from build123d import *

# Parameters (mm, degrees)
SKETCH1_R           = 1.513948887
SKETCH1_R_2         = 2.25
BOSS_EXTRUDE1_DEPTH = 2
SCALE1_SCALE        = 2.8


with BuildPart() as part:
    # Sketch1 → Boss-Extrude1 (new body)
    with BuildSketch(Plane.XY):
        with BuildLine():
            Line((-137.330840139, 84.740646997), (-129.065622639, 84.500215059))
            Line((-129.065622639, 84.500215059), (-129.094489584, 83.519353553))
            add(Edge.make_bspline(
                [(-129.094489584, 83.519353553), (-129.101127466, 83.291204798), (-129.199889222, 82.884598348), (-129.259340655, 82.689308143)],
                knots=[0.212765957, 0.212765957, 0.212765957, 0.212765957, 0.234042553, 0.234042553, 0.234042553, 0.234042553], degree=3))
            add(Edge.make_bspline(
                [(-129.259340655, 82.689308143), (-130.523557303, 78.537033893), (-136.295329969, 80.981325314), (-144.988370325, 77.341015795)],
                knots=[0.234042553, 0.234042553, 0.234042553, 0.234042553, 0.255319149, 0.255319149, 0.255319149, 0.255319149], degree=3))
            add(Edge.make_bspline(
                [(-144.988370325, 77.341015795), (-145.098029788, 77.295108948), (-145.047490899, 77.331606959), (-145.163209238, 77.309852904)],
                knots=[0.255319149, 0.255319149, 0.255319149, 0.255319149, 0.276595745, 0.276595745, 0.276595745, 0.276595745], degree=3))
            add(Edge.make_bspline(
                [(-145.163209238, 77.309852904), (-145.220654832, 77.299037913), (-145.285896319, 77.302718732), (-145.330562439, 77.26739941)],
                knots=[0.276595745, 0.276595745, 0.276595745, 0.276595745, 0.29787234, 0.29787234, 0.29787234, 0.29787234], degree=3))
            add(Edge.make_bspline(
                [(-145.330562439, 77.26739941), (-145.851667181, 76.854361866), (-147.089249586, 75.848112745), (-149.250531504, 76.047683454)],
                knots=[0.29787234, 0.29787234, 0.29787234, 0.29787234, 0.319148936, 0.319148936, 0.319148936, 0.319148936], degree=3))
            add(Edge.make_bspline(
                [(-149.250531504, 76.047683454), (-149.579241067, 76.078019194), (-149.46315051, 76.145142448), (-149.823167715, 76.007773448)],
                knots=[0.319148936, 0.319148936, 0.319148936, 0.319148936, 0.340425532, 0.340425532, 0.340425532, 0.340425532], degree=3))
            add(Edge.make_bspline(
                [(-149.823167715, 76.007773448), (-150.230952854, 75.852269176), (-150.642170668, 75.684998689), (-151.060274508, 75.505196874)],
                knots=[0.340425532, 0.340425532, 0.340425532, 0.340425532, 0.361702128, 0.361702128, 0.361702128, 0.361702128], degree=3))
            add(Edge.make_bspline(
                [(-151.060274508, 75.505196874), (-151.574575938, 75.284016862), (-153.203689978, 76.198038715), (-153.745700946, 75.937300235)],
                knots=[0.361702128, 0.361702128, 0.361702128, 0.361702128, 0.382978723, 0.382978723, 0.382978723, 0.382978723], degree=3))
            add(Edge.make_bspline(
                [(-153.745700946, 75.937300235), (-155.594836987, 75.047762033), (-159.716630745, 73.288289093), (-162.232470675, 71.858787121)],
                knots=[0.382978723, 0.382978723, 0.382978723, 0.382978723, 0.404255319, 0.404255319, 0.404255319, 0.404255319], degree=3))
            add(Edge.make_bspline(
                [(-162.232470675, 71.858787121), (-162.860836143, 71.501768336), (-162.462583912, 70.287097997), (-163.071821528, 69.816015174)],
                knots=[0.404255319, 0.404255319, 0.404255319, 0.404255319, 0.425531915, 0.425531915, 0.425531915, 0.425531915], degree=3))
            add(Edge.make_bspline(
                [(-163.071821528, 69.816015174), (-163.094733593, 69.798293477), (-163.120271861, 69.783446128), (-163.145313839, 69.766923799)],
                knots=[0.425531915, 0.425531915, 0.425531915, 0.425531915, 0.446808511, 0.446808511, 0.446808511, 0.446808511], degree=3))
            Line((-163.145313839, 69.766923799), (-163.880340349, 69.282192995))
            add(Edge.make_bspline(
                [(-163.880340349, 69.282192995), (-164.468258164, 68.894466252), (-164.620846731, 69.006028161), (-165.195757605, 69.192653966)],
                knots=[0.468085106, 0.468085106, 0.468085106, 0.468085106, 0.489361702, 0.489361702, 0.489361702, 0.489361702], degree=3))
            add(Edge.make_bspline(
                [(-165.195757605, 69.192653966), (-165.880330422, 69.414858475), (-166.586588499, 69.876830428), (-166.216843664, 70.149863853)],
                knots=[0.489361702, 0.489361702, 0.489361702, 0.489361702, 0.509556789, 0.509556789, 0.509556789, 0.509556789], degree=3))
            ThreePointArc((-166.216843664, 70.149863853), (-169.932333673, 71.346005011), (-168.915752591, 75.114583334))
            Line((-168.915752591, 75.114583334), (-169.065622639, 75.20554687))
            Line((-169.065622639, 75.20554687), (-169.064671417, 75.244319545))
            Line((-169.064671417, 75.244319545), (-169.037168666, 76.350054178))
            add(Edge.make_bspline(
                [(-169.037168666, 76.350054178), (-169.033053593, 76.794047826), (-168.700084206, 77.078711631), (-168.409216773, 77.250221263)],
                knots=[0.957446809, 0.957446809, 0.957446809, 0.957446809, 1, 1, 1, 1], degree=3))
            add(Edge.make_bspline(
                [(-168.409216773, 77.250221263), (-167.016522993, 78.071374807), (-166.193859899, 78.40091152), (-164.934151222, 79.073281388)],
                knots=[0, 0, 0, 0, 0.021276596, 0.021276596, 0.021276596, 0.021276596], degree=3))
            add(Edge.make_bspline(
                [(-164.934151222, 79.073281388), (-164.508106737, 79.300665029), (-163.405349845, 79.062094179), (-162.816253342, 79.349694368)],
                knots=[0.021276596, 0.021276596, 0.021276596, 0.021276596, 0.042553191, 0.042553191, 0.042553191, 0.042553191], degree=3))
            add(Edge.make_bspline(
                [(-162.816253342, 79.349694368), (-160.762294186, 80.3524281), (-156.1821764, 82.606350861), (-154.813800841, 83.397685633)],
                knots=[0.042553191, 0.042553191, 0.042553191, 0.042553191, 0.063829787, 0.063829787, 0.063829787, 0.063829787], degree=3))
            add(Edge.make_bspline(
                [(-154.813800841, 83.397685633), (-154.362548949, 83.658651579), (-154.360419036, 84.858143709), (-153.955446208, 85.0823635)],
                knots=[0.063829787, 0.063829787, 0.063829787, 0.063829787, 0.085106383, 0.085106383, 0.085106383, 0.085106383], degree=3))
            add(Edge.make_bspline(
                [(-153.955446208, 85.0823635), (-151.58212429, 86.396519351), (-151.052789401, 86.655893033), (-149.40636724, 86.835736205)],
                knots=[0.085106383, 0.085106383, 0.085106383, 0.085106383, 0.106382979, 0.106382979, 0.106382979, 0.106382979], degree=3))
            add(Edge.make_bspline(
                [(-149.40636724, 86.835736205), (-148.241325924, 86.963034649), (-146.873012401, 86.919588575), (-145.02819822, 86.765759283)],
                knots=[0.106382979, 0.106382979, 0.106382979, 0.106382979, 0.127659574, 0.127659574, 0.127659574, 0.127659574], degree=3))
            add(Edge.make_bspline(
                [(-145.02819822, 86.765759283), (-143.567802181, 86.644002746), (-141.759858228, 86.186588584), (-139.486373361, 85.727582157)],
                knots=[0.127659574, 0.127659574, 0.127659574, 0.127659574, 0.14893617, 0.14893617, 0.14893617, 0.14893617], degree=3))
            add(Edge.make_bspline(
                [(-139.486373361, 85.727582157), (-138.947939819, 85.618873917), (-138.058442974, 84.761801368), (-137.330840139, 84.740646997)],
                knots=[0.14893617, 0.14893617, 0.14893617, 0.14893617, 0.170212766, 0.170212766, 0.170212766, 0.170212766], degree=3))
        make_face()
        with Locations((-148.728458674, 81.356006962)):
            Circle(SKETCH1_R, mode=Mode.SUBTRACT)
        with Locations((-167.447114441, 72.697013944)):
            Circle(SKETCH1_R_2, mode=Mode.SUBTRACT)
    extrude(amount=BOSS_EXTRUDE1_DEPTH)


with BuildPart() as part_1:
    # Scale1: scaled about (-150.446524344, 79.751047586, 1)
    add(part.part.scale(SCALE1_SCALE).moved(Location((270.803743819, -143.551885655, -1.8))))


solid = part_1.part
Geometry: final body of the model. Coordinates: model frame, mm. Give positions to 0.01 mm unless a question says otherwise; leave off trailing zeros.
(1) Ray query, line 1 (X direction, y = 83, z = 0.95); line 2 (Y direction, x = -149, z = 1.55); line 3 (Y direction, x = -111, z = 2.1). Return the intervals inside material, ascending.
(2) Mould query, pull axis X, two halves, no side actions, for faces 1 (the flat face through (-147, 75, 3.8)), 2 (the cylindrical face through (-141.593, 85.518, 0.961)), 3 (the flat face through (-187.018, 51.126, 0.961)). Classes: released by +X, released by -X, zero draft, split by the parting line, or undercut.
(3) Cut plane A-A, the plane z = 2.1. Give the number of separate pieces and of enclosed holes in the cut face, then the cut area to 3 significant figures.
(4) First-contact query: P1, Ø7, axis at x = -145.64, y = 84.24, coming from the -Z side; P2, Ø1, axis at y = 82.5, z = 3, coming from the +X side. Flat tips, straight axial feed; report the tip coordinate or a pass-through.
Values follow:
1. line 1: x = -176.2 to -149.69, -141.58 to -94.63
1. line 2: y = 69.16 to 81.67, 86.82 to 99.4
1. line 3: y = 79.22 to 93.64
2. face 1: zero draft
2. face 2: undercut
2. face 3: released by +X
3. separate pieces: 1
3. enclosed holes: 2
3. area: 2,280 mm2
4. P1: passes through
4. P2: stops at x = -94.63
